Verification items for the finished model (mm, model axes). Face numbers are marked on the shaded views. A direction names the side the tool comes from. Coordinates: 2 decimals unless noted, no trailing zeros. Answer as a JSON object with one key per item and string values. Group by question number.
(1) Gauge pin test, flat ends, axial feed: pin 1 Ø5.5 at (y, z) = (14, -13.5) entering from +X (3 decimals); pin 2 Ø1.5 at (y, z) = (14, 14) entering from -X (3 decimals); pin 3 Ø8.5 at (x, y) = (-6, 16.5) entering from +Z. Record the tip position at first contact, or that the pin passes through.
(2) Cross-section at A-A (x = 0). Count the separate pieces of the cut face and the enclosed holes in it, plus the area to 3 significant figures.
(3) Material ranges on line 1 (Y direction, x = 0, z = 15.5) (1 decimal); line 2 (Y direction, x = -15, z = 4) (3 decimals); line 3 (Z direction, x = -8, y = 7), recorded low to high.
(4) Access from +Z, -Z, +X, -X, +Y, -Y to the whole of each face (thin tool, end or side, straight path). Record for the marked faces 5, 6 and 7.
(5) Mould release check, pull along X, two halves, no side actions. Record for the marked faces 1, 2, 3 and 4: released by +X, released by -X, zero draft, split by the parting line, or undercut.
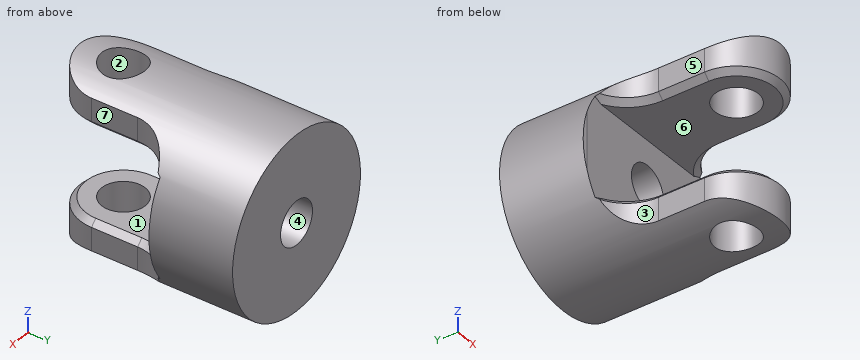
from build123d import *

# Parameters (mm, degrees)
SKETCH1_R               = 19.05
BASE_EXTRUDE_DEPTH      = 47.625
CUT_EXTRUDE1_DEPTH      = 55.716959208
CUT_EXTRUDE1_DEPTH_BACK = 55.716959208
CUT_EXTRUDE5_DEPTH      = 55.716959365
CUT_EXTRUDE5_DEPTH_BACK = 55.716959365
CUT_EXTRUDE6_DEPTH      = 55.716959365
CUT_EXTRUDE6_DEPTH_BACK = 55.716959365
SKETCH11_R              = 4.7625
SKETCH12_R              = 4.7625
CUT_EXTRUDE7_DEPTH      = 55.716959365
CHAMFER1_SIZE           = 1.27


with BuildPart() as part:
    # Sketch1 → Base-Extrude (new body)
    with BuildSketch(Plane(origin=(0, 0, 0), x_dir=(-1, 0, 0), z_dir=(0, 1, 0))):
        with Locations(Location((0, 0, 0), (0, 0, 90))):
            Circle(SKETCH1_R)
    extrude(amount=BASE_EXTRUDE_DEPTH)

    # Sketch2 → Cut-Extrude1 (cut, two sides: drawn at the far end of the back side and taken through both)
    with BuildSketch(Plane.XY.offset(-CUT_EXTRUDE1_DEPTH_BACK)):
        with BuildLine():
            Line((-19.05, -131.979516723), (-19.05, 0))
            Line((-19.05, 0), (-19.05, 29.21))
            ThreePointArc((-19.05, 29.21), (-12.314807909, 26.420192091), (-9.525, 19.685))
            Line((-9.525, 19.685), (-9.525, 9.525))
            ThreePointArc((-9.525, 9.525), (0, 0), (9.525, 9.525))
            Line((9.525, 9.525), (9.525, 19.685))
            ThreePointArc((9.525, 19.685), (12.314807909, 26.420192091), (19.05, 29.21))
            Line((19.05, 29.21), (19.05, 0))
            Line((19.05, 0), (19.05, -131.979516723))
            Line((19.05, -131.979516723), (19.05, -395.938550169))
            Line((19.05, -395.938550169), (-19.05, -395.938550169))
            Line((-19.05, -395.938550169), (-19.05, -131.979516723))
        make_face()
    extrude(amount=CUT_EXTRUDE1_DEPTH + CUT_EXTRUDE1_DEPTH_BACK, mode=Mode.SUBTRACT)

    # Sketch8 → Cut-Extrude5 (cut, two sides: drawn at the far end of the back side and taken through both)
    with BuildSketch(Plane(origin=(0, 0, 0), x_dir=(0, 0, -1), z_dir=(1, 0, 0)).offset(-CUT_EXTRUDE5_DEPTH_BACK)):
        Polygon((-10.16, -121.738350451), (-10.16, 0), (-10.16, 29.145238826), (10.16, 29.145238826), (10.16, 0), (10.16, -121.738350451), (10.16, -365.215051352), (-10.16, -365.215051352), align=None)
    extrude(amount=CUT_EXTRUDE5_DEPTH + CUT_EXTRUDE5_DEPTH_BACK, mode=Mode.SUBTRACT)

    # Sketch11 → Cut-Extrude6 (cut, two sides: drawn at the far end of the back side and taken through both)
    with BuildSketch(Plane.XY.offset(-CUT_EXTRUDE6_DEPTH_BACK)):
        with Locations(Location((0, 9.525, 0), (0, 0, 90))):
            Circle(SKETCH11_R)
    extrude(amount=CUT_EXTRUDE6_DEPTH + CUT_EXTRUDE6_DEPTH_BACK, mode=Mode.SUBTRACT)

    # Sketch12 → Cut-Extrude7 (cut, through all)
    with BuildSketch(Plane(origin=(0, 47.625, 0), x_dir=(-1, 0, 0), z_dir=(0, 1, 0))):
        with Locations(Location((0, 0, 0), (0, 0, 90))):
            Circle(SKETCH12_R)
    extrude(amount=-CUT_EXTRUDE7_DEPTH, mode=Mode.SUBTRACT)

    # Chamfer1
    # the kernel refuses this chamfer: 1.27 mm, written as the material it takes off along each edge
    with BuildSketch(Plane(origin=(19.05, 19.685, -10.16), x_dir=(-1, 0, 0), z_dir=(0, -1, 0))) as chamfer1_piece_1_section:
        Polygon((9.525 + CHAMFER1_SIZE, 0), (9.525, CHAMFER1_SIZE), (9.525, 0), align=None)
    chamfer1_piece_1 = revolve(axis=Axis((19.05, 19.685, -10.16), (0, 0, -1)), revolution_arc=91.701103325, mode=Mode.PRIVATE)
    chamfer1_piece_1 = split(chamfer1_piece_1, bisect_by=Plane(origin=(9.159628587, 29.145238826, -10.520330591), z_dir=(0, -1, 0)), keep=Keep.TOP, mode=Mode.PRIVATE)
    add(chamfer1_piece_1, mode=Mode.SUBTRACT)
    with BuildSketch(Plane(origin=(9.525, 19.685, -10.16), x_dir=(-0.9996219169112966, 0, 0.027495876610585942), z_dir=(0, -1, 0)), Plane(origin=(-9.525, 9.525, -10.16), x_dir=(0.9996219169112966, 0, 0.027495876610585942), z_dir=(0, 1, 0)), Plane(origin=(-9.525, 19.685, 10.16), x_dir=(0.9996219169112966, 0, -0.027495876610585942), z_dir=(0, -1, 0))) as chamfer1_piece_2:
        Polygon((CHAMFER1_SIZE * 0.999621916911, CHAMFER1_SIZE * 0.0274958766106), (-CHAMFER1_SIZE * 0.0274958766106, CHAMFER1_SIZE * 0.999621916911), (0, 0), align=None)
    extrude(amount=10.16, mode=Mode.SUBTRACT)
    with BuildSketch(Plane(origin=(0, 9.525, -10.16), x_dir=(1, 0, 0), z_dir=(0, 1, 0))) as chamfer1_piece_3:
        Polygon((9.525 - CHAMFER1_SIZE, 0), (9.525, CHAMFER1_SIZE), (9.525, 0), align=None)
    revolve(axis=Axis((0, 9.525, -10.16), (0, 0, -1)), revolution_arc=180, mode=Mode.SUBTRACT)
    with BuildSketch(Plane(origin=(-19.05, 19.685, -10.16), x_dir=(-0.029685492056236547, 0.9995592886674503, 0), z_dir=(-0.9995592886674503, -0.029685492056236547, 0))) as chamfer1_piece_4_section:
        Polygon((9.525 + CHAMFER1_SIZE, 0), (9.525, CHAMFER1_SIZE), (9.525, 0), align=None)
    chamfer1_piece_4 = revolve(axis=Axis((-19.05, 19.685, -10.16), (0, 0, -1)), revolution_arc=91.701103313, mode=Mode.PRIVATE)
    chamfer1_piece_4 = split(chamfer1_piece_4, bisect_by=Plane(origin=(-11.981482464, 29.145238826, -10.596388044), z_dir=(0, -1, 0)), keep=Keep.TOP, mode=Mode.PRIVATE)
    add(chamfer1_piece_4, mode=Mode.SUBTRACT)
    with BuildSketch(Plane(origin=(19.05, 19.685, 10.16), x_dir=(-1, 0, 0), z_dir=(0, -1, 0))) as chamfer1_piece_5_section:
        Polygon((9.525, -CHAMFER1_SIZE), (9.525 + CHAMFER1_SIZE, 0), (9.525, 0), align=None)
    chamfer1_piece_5 = revolve(axis=Axis((19.05, 19.685, 10.16), (0, 0, -1)), revolution_arc=91.701103313, mode=Mode.PRIVATE)
    chamfer1_piece_5 = split(chamfer1_piece_5, bisect_by=Plane(origin=(11.981482474, 29.145238826, 10.59638804), z_dir=(0, -1, 0)), keep=Keep.TOP, mode=Mode.PRIVATE)
    add(chamfer1_piece_5, mode=Mode.SUBTRACT)
    with BuildSketch(Plane(origin=(9.525, 9.525, 10.16), x_dir=(0.02749587661058595, 0, 0.9996219169112968), z_dir=(0, 1, 0))) as chamfer1_piece_6:
        Polygon((CHAMFER1_SIZE * 0.999621916911, -CHAMFER1_SIZE * 0.0274958766106), (-CHAMFER1_SIZE * 0.0274958766106, -CHAMFER1_SIZE * 0.999621916911), (0, 0), align=None)
    extrude(amount=10.16, mode=Mode.SUBTRACT)
    with BuildSketch(Plane(origin=(0, 9.525, 10.16), x_dir=(1, 0, 0), z_dir=(0, 1, 0))) as chamfer1_piece_7:
        Polygon((9.525, -CHAMFER1_SIZE), (9.525 - CHAMFER1_SIZE, 0), (9.525, 0), align=None)
    revolve(axis=Axis((0, 9.525, 10.16), (0, 0, -1)), revolution_arc=180, mode=Mode.SUBTRACT)
    with BuildSketch(Plane(origin=(-19.05, 19.685, 10.16), x_dir=(-0.02968549226478587, 0.9995592886612565, 0), z_dir=(-0.9995592886612565, -0.02968549226478587, 0))) as chamfer1_piece_8_section:
        Polygon((9.525 + CHAMFER1_SIZE, 0), (9.525, -CHAMFER1_SIZE), (9.525, 0), align=None)
    chamfer1_piece_8 = revolve(axis=Axis((-19.05, 19.685, 10.16), (0, 0, -1)), revolution_arc=91.701103325, mode=Mode.PRIVATE)
    chamfer1_piece_8 = split(chamfer1_piece_8, bisect_by=Plane(origin=(-11.981482467, 29.145238826, 10.596388044), z_dir=(0, -1, 0)), keep=Keep.TOP, mode=Mode.PRIVATE)
    add(chamfer1_piece_8, mode=Mode.SUBTRACT)


solid = part.part
Taken from the geometry:
{
 "1": {"pin 1": "stops at x = 9.525", "pin 2": "stops at x = -9.525", "pin 3": "stops at z = 18.97"},
 "2": {"separate pieces": "4", "enclosed holes": "0", "area": "875 mm²"},
 "3": {"line 1": "y = 0 to 4.8, 14.3 to 47.6", "line 2": "y = 29.145 to 47.625", "line 3": "z = -17.29 to -10.29, 10.29 to 17.29"},
 "4": {"face 5": "+Z, -Z, -X, -Y", "face 6": "+X, -X, -Y", "face 7": "+Z, -Z, +X, -Y"},
 "5": {"face 1": "zero draft", "face 2": "undercut", "face 3": "released by -X", "face 4": "undercut"}
}
